The model under review builds one solid part; all positions refer to its coordinate system, in mm. Face numbers are marked on the shaded views. A direction names the side the tool comes from. Round coordinates to 2 decimals unless told otherwise and drop trailing zeros. Loops run counter-clockwise (first coordinate to the right, second up) from the corner with the lowest first, then second, coordinate; pieces in that order, holes last. Notation, with made-up numbers: M -11.75,58.25 L 28.25,58.25 A32 ccw 28.25,90.25 Z; hole C -35.75,86 d10. An arc over 180 degrees is marked long. Use a Markdown table: item, result. Add a question column.
```python
from build123d import *

# Parameters (mm, degrees)
SKETCH_1_W          = 2.85
SKETCH_1_H          = 1.1
SKETCH_2_W          = 0.5
SKETCH_2_H          = 0.5
EXTRUDE_1_DEPTH     = 1.2
SKETCH_3_W          = 0.5
SKETCH_3_H          = 0.5
EXTRUDE_2_DEPTH     = 1.2
SKETCH_4_R          = 2.45
EXTRUDE_3_DEPTH     = 4.4
FILLET_1_R          = 0.1
CUT_EXTRUDE_1_DEPTH = 0.3
SKETCH_7_R          = 0.071568043
SKETCH_7_R_2        = 0.102987613
CUT_EXTRUDE_2_DEPTH = 1


with BuildPart() as part:
    # 草图1 → 旋转1 (revolve)
    with BuildSketch(Plane.XY, mode=Mode.PRIVATE) as revolve_1_sk:
        with Locations((1.425, 0.55)):
            Rectangle(SKETCH_1_W, SKETCH_1_H)
    revolve(revolve_1_sk.sketch.rotate(Axis((0, 1.1, 0), (0, -1, 0)), 270), axis=Axis((0, 1.1, 0), (0, -1, 0)))

    # 草图2 → 凸台-拉伸1 (add)
    with BuildSketch(Plane.XZ):
        with Locations((1.27, 0)):
            Rectangle(SKETCH_2_W, SKETCH_2_H)
    extrude(amount=EXTRUDE_1_DEPTH)

    # 草图3 → 凸台-拉伸2 (add)
    with BuildSketch(Plane.XZ):
        with Locations((-1.27, 0)):
            Rectangle(SKETCH_3_W, SKETCH_3_H)
    extrude(amount=EXTRUDE_2_DEPTH)

    # 草图4 → 凸台-拉伸3 (add)
    with BuildSketch(Plane(origin=(0, 1.1, 0), x_dir=(-1, 0, 0), z_dir=(0, 1, 0))):
        with Locations(Location((0, 0, 0), (0, 0, 90))):
            Circle(SKETCH_4_R)
    extrude(amount=EXTRUDE_3_DEPTH)

    # 圆角1
    fillet_1_edges = [part.edges().sort_by_distance(p)[0] for p in [
        (0, 5.5, -2.45),
    ]]
    fillet(fillet_1_edges, radius=FILLET_1_R)

    # 草图6 → 切除-拉伸1 (cut, symmetric)
    with BuildSketch(Plane.XY):
        Polygon((-1.02, 3.852964397), (-0.181256176, 3.852964397), (-1.27, 4.752964397), (-1.27, 3.852964397), (-1.52, 3.852964397), (-1.52, 0.252964397), (-1.02, 0.252964397), align=None)
        Polygon((1.52, 0.252964397), (1.02, 0.252964397), (1.02, 3.516785867), (-0.475424156, 4.752964397), (1.52, 4.752964397), align=None)
    extrude(amount=CUT_EXTRUDE_1_DEPTH, both=True, mode=Mode.SUBTRACT)

    # 草图7 → 切除-拉伸2 (cut)
    with BuildSketch(Plane.XZ.offset(1.2)):
        with Locations(Location((-1.27, 0, 0), (0, 0, 270))):
            Circle(SKETCH_7_R)
        with Locations(Location((1.27, 0, 0), (0, 0, 270))):
            Circle(SKETCH_7_R_2)
    extrude(amount=-CUT_EXTRUDE_2_DEPTH, mode=Mode.SUBTRACT)


solid = part.part
```
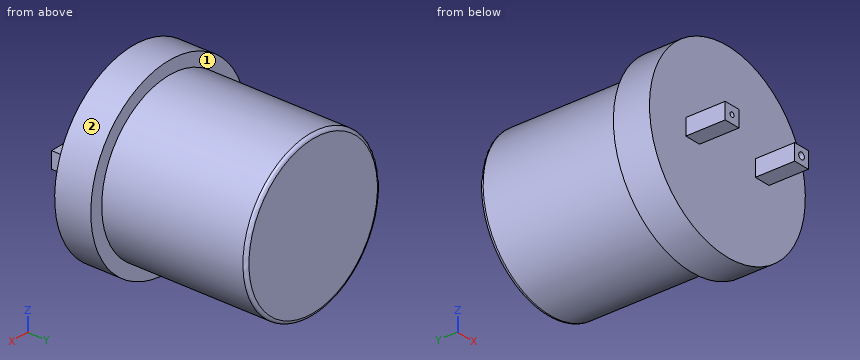
(1) Insertion check: pin 1 Ø2 at (x, z) = (-2, -2) entering from -Y; pin 2 Ø3 at (y, z) = (3, -0.5) entering from +X; pin 3 Ø1.6 at (x, y) = (0.5, 2.5) entering from +Z; pin 4 Ø0.7 at (x, z) = (1, 0) entering from -Y. Each pin has a flat end and moves straight along its axis. Give the tip position at first contact, or say it passes through.
(2) Consider section B-B, the plane y = 5.25. Give the boundary of the cut face in (x, z), then the cut area to 3 significant figures.
(3) Consider section D-D, the plane x = 2.55. Give the boundary of the cut face in (y, z), then the cut area to 3 significant figures.
(4) For the marked faces 1 and 2, list the 3-axis set-ups (+Z, -Z, +X, -X, +Y, -Y) from which the entire face can be reached by the end or side of a thin tool; tool diameter is ignored.
(5) To check wall thickness, follow probe 1 along Z at (x, y) = (0.05, 1.5); probe 2 along Y at (x, z) = (-2.2, -0.35); probe 3 along Y at (x, z) = (1.25, 2.25). State the ranges of each line that lie inside material, in increasing order.
(6) Consider section A-A, the plane y = 1.5. Give the boundary of the cut face in (x, z).
(7) Consider section C-C, the plane x = -0.3. Give the number of separate pieces and of enclosed holes in the cut face, then the cut area to 3 significant figures.
Found:
| question | item | result |
|---|---|---|
| 1 | pin 1 | stops at y = 0 |
| 1 | pin 2 | stops at x = 2.45 |
| 1 | pin 3 | stops at z = 2.45 |
| 1 | pin 4 | stops at y = -1.2 |
| 2 | outline | C 0,0 d4.9 |
| 2 | area | 18.9 mm^2 |
| 3 | outline | M 0,-1.27 L 1.1,-1.27 L 1.1,1.27 L 0,1.27 Z |
| 3 | area | 2.80 mm^2 |
| 4 | face 1 | +Y |
| 4 | face 2 | +Y, -Y |
| 5 | probe 1 | z = -2.45 to 2.45 |
| 5 | probe 2 | y = 0 to 5.5 |
| 5 | probe 3 | y = 0 to 1.1 |
| 6 | outline | C 0,0 d4.9; hole M -1.52,-0.3 L -1.02,-0.3 L -1.02,0.3 L -1.52,0.3 Z; hole M 1.02,-0.3 L 1.52,-0.3 L 1.52,0.3 L 1.02,0.3 Z |
| 7 | separate pieces | 1 |
| 7 | enclosed holes | 2 |
| 7 | area | 27.5 mm^2 |
